Could you check a few things on this model? Use its own coordinates, in mm. A direction names the side the tool comes from. Give positions to 0.01 mm unless a question says otherwise; leave off trailing zeros. Order: outer loops, then holes, each group sorted by start corner. A loop starts at its lowest first (then second) coordinate and runs counter-clockwise, first axis right, second up. Notation, with made-up numbers: (-32, -3) - (-8, -3) arc R18 ccw to (-8, 27) - close; hole circle Ø1 at (45, 33.25). An arc over 180 degrees is marked (long way). One line per question, with ' | ' between items. Start each with the question number.
1. Imagine slicing it at A-A (x = 15). Please give me the cut outline in (y, z), and give its area (3 significant figures).
2. Which directions (+Z, -Z, +X, -X, +Y, -Y) give clear straight access to the entire face, cutting with the end or side of a thin tool? Please do faces 1 (the flat face through (30, 0, 2)), 2 (the flat face through (38, -18, 4.5)), 3 (the cylindrical face through (-15.521, -19.041, 3.534)).
3. If we mould it in two halves opening along X, with no side actions, what happens to faces 4 (the cylindrical face through (43.5, 26.07, 7.6)), 5 (the cylindrical face through (-43.57, 26, 7.6)), 6 (the flat face through (-39, 0, 12))? For each: released by +X, released by -X, zero draft, split by the parting line, or undercut.
4. For P1, Ø2.5, axis at y = -0.5, z = 6.5, coming from the -X side; P2, Ø5, axis at x = 36, y = 18.5, coming from the +Z side, each with a flat end and sliding along its axis, tell me the tip position at first contact or that it passes through.
5. I need wall thicknesses on probe 1 along Y at (x, z) = (36, 7.5); probe 2 along Y at (x, z) = (36, 3.3); probe 3 along X at (y, z) = (-24.25, 7.5). Which ranges of each line are inside material? Lowest first, please. Write a range as from..to.
6. Imagine slicing it at C-C (y = 10.5). Please give me the cut outline in (x, z), and give its area (3 significant figures).
7. Imagine slicing it at B-B (x = 28.5). Please give me the cut outline in (y, z).
8. Imagine slicing it at D-D (z = 2). Please give me the cut outline in (x, y).
```python
from build123d import *

# Parameters (mm, degrees)
SKETCH1_W                       = 90
SKETCH1_H                       = 55
BOSS_EXTRUDE1_DEPTH             = 15
SKETCH2_W                       = 60
SKETCH2_H                       = 25
CUT_EXTRUDE1_DEPTH              = 55.829280499
CBORE_FOR_M3_SBHCS1_D           = 3.4
CBORE_FOR_M3_SBHCS1_CBORE_D     = 8
CBORE_FOR_M3_SBHCS1_CBORE_DEPTH = 10.5
FILLET7_R                       = 5
FILLET8_R                       = 5
FILLET9_R                       = 5
FILLET10_R                      = 5
CBORE_FOR_M3_SBHCS2_D           = 3.4
CBORE_FOR_M3_SBHCS2_DEPTH       = 15
CBORE_FOR_M3_SBHCS2_CBORE_D     = 8
CBORE_FOR_M3_SBHCS2_CBORE_DEPTH = 10.5
CBORE_FOR_M3_SBHCS6_D           = 3.4
CBORE_FOR_M3_SBHCS6_DEPTH       = 15
CBORE_FOR_M3_SBHCS6_CBORE_D     = 8
CBORE_FOR_M3_SBHCS6_CBORE_DEPTH = 10.5
CBORE_FOR_M3_SBHCS7_D           = 3.4
CBORE_FOR_M3_SBHCS7_DEPTH       = 15
CBORE_FOR_M3_SBHCS7_CBORE_D     = 8
CBORE_FOR_M3_SBHCS7_CBORE_DEPTH = 10.5
CBORE_FOR_M3_SBHCS8_D           = 3.4
CBORE_FOR_M3_SBHCS8_DEPTH       = 15
CBORE_FOR_M3_SBHCS8_CBORE_D     = 8
CBORE_FOR_M3_SBHCS8_CBORE_DEPTH = 10.5
CHAMFER5_SIZE                   = 12
CHAMFER7_SIZE                   = 12
CHAMFER8_SIZE                   = 12
CHAMFER9_SIZE                   = 12


with BuildPart() as part:
    # Sketch1 → Boss-Extrude1 (new body)
    with BuildSketch(Plane.XY):
        Rectangle(SKETCH1_W, SKETCH1_H)
    extrude(amount=BOSS_EXTRUDE1_DEPTH)

    # Sketch2 → Cut-Extrude1 (cut, through all)
    with BuildSketch(Plane.XY.offset(15)):
        Rectangle(SKETCH2_W, SKETCH2_H)
    extrude(amount=-CUT_EXTRUDE1_DEPTH, mode=Mode.SUBTRACT)

    # CBORE for M3 SBHCS1 (through all)
    with Locations(Plane.XY.offset(15)):
        with Locations((-36, -18.5), (-36, 18.5), (36, 18.5), (36, -18.5)):
            CounterBoreHole(CBORE_FOR_M3_SBHCS1_D / 2, CBORE_FOR_M3_SBHCS1_CBORE_D / 2, CBORE_FOR_M3_SBHCS1_CBORE_DEPTH)

    # Fillet7
    fillet7_edges = [part.edges().sort_by_distance(p)[0] for p in [
        (-45, -27.5, 7.5),
    ]]
    fillet(fillet7_edges, radius=FILLET7_R)

    # Fillet8
    fillet8_edges = [part.edges().sort_by_distance(p)[0] for p in [
        (-45, 27.5, 7.5),
    ]]
    fillet(fillet8_edges, radius=FILLET8_R)

    # Fillet9
    fillet9_edges = [part.edges().sort_by_distance(p)[0] for p in [
        (45, 27.5, 7.5),
    ]]
    fillet(fillet9_edges, radius=FILLET9_R)

    # Fillet10
    fillet10_edges = [part.edges().sort_by_distance(p)[0] for p in [
        (45, -27.5, 7.5),
    ]]
    fillet(fillet10_edges, radius=FILLET10_R)

    # CBORE for M3 SBHCS2
    with Locations(Plane(origin=(-30, 0, 0), x_dir=(0, 0, -1), z_dir=(1, 0, 0))):
        with Locations((-7.5, 0)):
            CounterBoreHole(CBORE_FOR_M3_SBHCS2_D / 2, CBORE_FOR_M3_SBHCS2_CBORE_D / 2, CBORE_FOR_M3_SBHCS2_CBORE_DEPTH, depth=CBORE_FOR_M3_SBHCS2_DEPTH)

    # CBORE for M3 SBHCS6
    with Locations(Plane(origin=(0, -12.5, 0), x_dir=(1, 0, 0), z_dir=(0, 1, 0))):
        with Locations((-15, -7.5), (15, -7.5)):
            CounterBoreHole(CBORE_FOR_M3_SBHCS6_D / 2, CBORE_FOR_M3_SBHCS6_CBORE_D / 2, CBORE_FOR_M3_SBHCS6_CBORE_DEPTH, depth=CBORE_FOR_M3_SBHCS6_DEPTH)

    # CBORE for M3 SBHCS7
    with Locations(Plane(origin=(0, 12.5, 0), x_dir=(-1, 0, 0), z_dir=(0, -1, 0))):
        with Locations((15, -7.5), (-15, -7.5)):
            CounterBoreHole(CBORE_FOR_M3_SBHCS7_D / 2, CBORE_FOR_M3_SBHCS7_CBORE_D / 2, CBORE_FOR_M3_SBHCS7_CBORE_DEPTH, depth=CBORE_FOR_M3_SBHCS7_DEPTH)

    # CBORE for M3 SBHCS8
    with Locations(Plane.ZY.offset(-30)):
        with Locations((7.5, 0)):
            CounterBoreHole(CBORE_FOR_M3_SBHCS8_D / 2, CBORE_FOR_M3_SBHCS8_CBORE_D / 2, CBORE_FOR_M3_SBHCS8_CBORE_DEPTH, depth=CBORE_FOR_M3_SBHCS8_DEPTH)

    # Chamfer5
    # the kernel refuses this chamfer: 12 mm, written as the material it takes off along each edge
    with BuildSketch(Plane(origin=(30, 12.5, 15), x_dir=(0, -0.027495876610586348, -0.9996219169112968), z_dir=(-1, 0, 0))) as chamfer5_piece_1:
        Polygon((CHAMFER5_SIZE * 0.999621916911, -CHAMFER5_SIZE * 0.0274958766106), (-CHAMFER5_SIZE * 0.0274958766106, -CHAMFER5_SIZE * 0.999621916911), (0, 0), align=None)
    extrude(amount=60, mode=Mode.SUBTRACT)

    # Chamfer7
    # the kernel refuses this chamfer: 12 mm, written as the material it takes off along each edge
    with BuildSketch(Plane(origin=(-30, -12.5, 15), x_dir=(0, -0.9996219169112969, 0.027495876610586348), z_dir=(1, 0, 0))) as chamfer7_piece_1:
        Polygon((CHAMFER7_SIZE * 0.999621916911, CHAMFER7_SIZE * 0.0274958766106), (-CHAMFER7_SIZE * 0.0274958766106, CHAMFER7_SIZE * 0.999621916911), (0, 0), align=None)
    extrude(amount=60, mode=Mode.SUBTRACT)

    # Chamfer8
    # the kernel refuses this chamfer: 12 mm, written as the material it takes off along each edge
    with BuildSketch(Plane(origin=(30, -55.360195856, 15), x_dir=(0.9996219169112969, 5.384635157726403e-15, 0.027495876610586355), z_dir=(0, 1, 0))) as chamfer8_piece_1_section:
        Polygon((CHAMFER8_SIZE * 0.999621916911, CHAMFER8_SIZE * 0.0274958766106), (-CHAMFER8_SIZE * 0.0274958766106, CHAMFER8_SIZE * 0.999621916911), (0, 0), align=None)
    chamfer8_piece_1 = extrude(amount=110.720391711, mode=Mode.PRIVATE)
    chamfer8_piece_1 = split(chamfer8_piece_1, bisect_by=Plane(origin=(33.163106807, 2.674956812, -6.825043188), z_dir=(0, -0.7071067811862648, 0.7071067811868302)), keep=Keep.TOP, mode=Mode.PRIVATE)
    chamfer8_piece_1 = split(chamfer8_piece_1, bisect_by=Plane(origin=(33.163106807, -18.33806362, 8.83806362), z_dir=(0, 0.7071067811868302, 0.7071067811862648)), keep=Keep.TOP, mode=Mode.PRIVATE)
    add(chamfer8_piece_1, mode=Mode.SUBTRACT)

    # Chamfer9
    # the kernel refuses this chamfer: 12 mm, written as the material it takes off along each edge
    with BuildSketch(Plane(origin=(-30, 55.360195856, 15), x_dir=(-0.9996219169112969, 5.384635157726403e-15, 0.027495876610586355), z_dir=(0, -1, 0))) as chamfer9_piece_1_section:
        Polygon((CHAMFER9_SIZE * 0.999621916911, CHAMFER9_SIZE * 0.0274958766106), (-CHAMFER9_SIZE * 0.0274958766106, CHAMFER9_SIZE * 0.999621916911), (0, 0), align=None)
    chamfer9_piece_1 = extrude(amount=110.720391711, mode=Mode.PRIVATE)
    chamfer9_piece_1 = split(chamfer9_piece_1, bisect_by=Plane(origin=(-33.163106802, 18.338063618, 8.838063618), z_dir=(0, -0.7071067811862648, 0.7071067811868302)), keep=Keep.TOP, mode=Mode.PRIVATE)
    chamfer9_piece_1 = split(chamfer9_piece_1, bisect_by=Plane(origin=(-33.163106802, -2.674956815, -6.825043185), z_dir=(0, 0.7071067811868302, 0.7071067811862648)), keep=Keep.TOP, mode=Mode.PRIVATE)
    add(chamfer9_piece_1, mode=Mode.SUBTRACT)


solid = part.part
```
Results found:
1) outline: (-27.5, 0) - (-12.5, 0) - (-12.5, 3) - (-13, 3.5) - (-23, 3.5) - (-23, 5.8) - (-27.5, 5.8) - close; (-27.5, 9.2) - (-23, 9.2) - (-23, 11.5) - (-21, 11.5) - (-24.5, 15) - (-27.5, 15) - close; (12.5, 0) - (27.5, 0) - (27.5, 5.8) - (23, 5.8) - (23, 3.5) - (13, 3.5) - (12.5, 3) - close; (21, 11.5) - (23, 11.5) - (23, 9.2) - (27.5, 9.2) - (27.5, 15) - (24.5, 15) - close | area: 179 mm2
2) face 1: +Z, -Z | face 2: +Z | face 3: none
3) face 4: released by +X | face 5: released by -X | face 6: undercut
4) P1: stops at x = -45 | P2: stops at z = 4.5
5) probe 1: y = -27.5..-22.5, -14.5..-4, 4..14.5, 22.5..27.5 | probe 2: y = -27.5..-20.2, -16.8..16.8, 20.2..27.5 | probe 3: x = -44.68..-16.7, -13.3..13.3, 16.7..44.68
6) outline: (-45, 0) - (-30, 0) - (-30, 3) - (-42, 15) - (-45, 15) - close; (30, 0) - (45, 0) - (45, 15) - (42, 15) - (30, 3) - close | area: 306 mm2
7) outline: (-27.5, 0) - (-12.5, 0) - (-12.5, 3) - (-24.5, 15) - (-27.5, 15) - close; (12.5, 0) - (27.5, 0) - (27.5, 15) - (24.5, 15) - (12.5, 3) - close
8) outline: (-45, -22.5) arc R5 ccw to (-40, -27.5) - (40, -27.5) arc R5 ccw to (45, -22.5) - (45, 22.5) arc R5 ccw to (40, 27.5) - (-40, 27.5) arc R5 ccw to (-45, 22.5) - close; hole circle Ø3.4 at (-36, -18.5); hole circle Ø3.4 at (-36, 18.5); hole (-30, -12.5) - (30, -12.5) - (30, 12.5) - (-30, 12.5) - close; hole circle Ø3.4 at (36, -18.5); hole circle Ø3.4 at (36, 18.5)
